```python
from build123d import *

# Parameters (mm, degrees)
F0_W     = 50
F0_H     = 100
F1_DEPTH = 12
F3_D     = 2.4
F3_DEPTH = 6
F3_TIP   = 0.7210327428
F5_D     = 2.4
F5_DEPTH = 6
F5_TIP   = 0.7210327428
F7_D     = 2.4
F7_DEPTH = 6
F7_TIP   = 0.7210327428
F9_D     = 2.4
F9_DEPTH = 6
F9_TIP   = 0.7210327428


with BuildPart() as f1:
    # F0 (on Top) → F1 (new body)
    with BuildSketch(Plane.XY):
        Rectangle(F0_W, F0_H)
    extrude(amount=F1_DEPTH)

    # F3
    with Locations(Plane.XY.offset(12)):
        with Locations((0, 20), (0, -20)):
            Hole(F3_D / 2, depth=F3_DEPTH)
            with Locations((0, 0, -(F3_DEPTH + F3_TIP / 2))):  # 118° drill point
                Cone(0, F3_D / 2, F3_TIP, mode=Mode.SUBTRACT)

    # F5
    with Locations(Plane.YZ.offset(25)):
        with Locations((-35, 6), (35, 6)):
            Hole(F5_D / 2, depth=F5_DEPTH)
            with Locations((0, 0, -(F5_DEPTH + F5_TIP / 2))):  # 118° drill point
                Cone(0, F5_D / 2, F5_TIP, mode=Mode.SUBTRACT)

    # F7
    with Locations(Plane(origin=(-25, 0, 0), x_dir=(0, -1, 0), z_dir=(-1, 0, 0))):
        with Locations((-35, 6), (35, 6)):
            Hole(F7_D / 2, depth=F7_DEPTH)
            with Locations((0, 0, -(F7_DEPTH + F7_TIP / 2))):  # 118° drill point
                Cone(0, F7_D / 2, F7_TIP, mode=Mode.SUBTRACT)

    # F9
    with Locations(Plane.XY.offset(12)):
        with Locations((-20, -45), (-20, 45)):
            Hole(F9_D / 2, depth=F9_DEPTH)
            with Locations((0, 0, -(F9_DEPTH + F9_TIP / 2))):  # 118° drill point
                Cone(0, F9_D / 2, F9_TIP, mode=Mode.SUBTRACT)


solid = f1.part
```
Work out the finished part from the listing and answer in its coordinate system (mm). A direction names the side the tool comes from. Coordinates: 2 decimals unless noted, no trailing zeros.
1) Flat-ended cylindrical pins translate along their axes: pin 1 (1.9 mm diameter, centred on x = 0, y = -20, fed in from +Z); pin 2 (3 mm diameter, centred on y = 35, z = 6, fed in from +X); pin 3 (2 mm diameter, centred on y = -35, z = 6, fed in from -X). Find the tip coordinate at first contact, or state that the pin passes through.
Results:
pin 1: stops at z = 5.85
pin 2: stops at x = 25
pin 3: stops at x = -18.88
2) For faces 1 (the cylindrical face through (21.96, 33.89, 5.54)), 2 (the flat face through (0, 1, 12)), 3 (the cylindrical face through (0.26, -21.17, 8.96)), 4 (the cylindrical face through (-21.96, -33.89, 5.54)), 5 (the flat face through (-25, -1, 6)), determine the directions among +Z, -Z, +X, -X, +Y, -Y from which every point of the face is accessible in a straight line to the end or side of a thin tool.
Results:
face 1: +X
face 2: +Z, +X, -X, +Y, -Y
face 3: +Z
face 4: -X
face 5: +Z, -Z, -X, +Y, -Y
3) For a pull along Z with two mould halves and no side action, classify faces 6 (the conical face through (18.404, 34.835, 5.873)), 7 (the conical face through (0.096, 19.815, 5.404)), 8 (the flat face through (0, -50, 6)) as +Z half, -Z half, draft (parallel to the pull), parting line (faces both ways), or undercut.
Results:
face 6: undercut
face 7: +Z half
face 8: draft
4) Consider probe 1 along Y at (x, z) = (0, 7.75); probe 2 along Y at (x, z) = (-21.8, 6); probe 3 along Z at (x, y) = (20.75, 35). Determine where each line is inside the solid, lowest interval first.
Results:
probe 1: y = -50 to -21.2, -18.8 to 18.8, 21.2 to 50
probe 2: y = -50 to -36.2, -33.8 to 33.8, 36.2 to 50
probe 3: z = 0 to 4.8, 7.2 to 12
